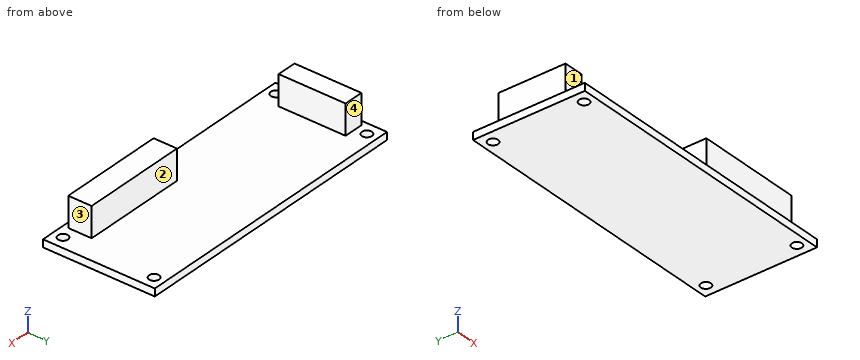
```python
from build123d import *

# Parameters (mm, degrees)
SKETCH1_W               = 91.44
SKETCH1_H               = 35.56
BOSS_EXTRUDE1_DEPTH     = 2.38125
SKETCH2_R               = 1.5875
CUT_EXTRUDE1_DEPTH      = 50.113309312
MIRROR2_COPY_1_SKETCH_R = 1.5875
MIRROR2_COPY_1_DEPTH    = 50.113309312
SKETCH3_W               = 6.208251033
SKETCH3_H               = 21.285432112
SKETCH3_W_2             = 33.591072552
SKETCH3_H_2             = 7.427728914
BOSS_EXTRUDE2_DEPTH     = 9.525


with BuildPart() as part:
    # Sketch1 → Boss-Extrude1 (new body)
    with BuildSketch(Plane.XY):
        Rectangle(SKETCH1_W, SKETCH1_H)
    extrude(amount=BOSS_EXTRUDE1_DEPTH)

    # Sketch2 → Cut-Extrude1 (cut, through all)
    with BuildSketch(Plane.XY.offset(2.38125)):
        with Locations((-41.91, 14.478)):
            Circle(SKETCH2_R)
    cut_extrude1 = extrude(amount=-CUT_EXTRUDE1_DEPTH, mode=Mode.SUBTRACT)

    # Mirror1: Cut-Extrude1 across plane
    add(cut_extrude1.mirror(Plane(origin=(0, 0, 0), x_dir=(0, 0, 1), z_dir=(1, 0, 0))), mode=Mode.SUBTRACT)

    # Mirror2: Cut-Extrude1 across plane
    add(cut_extrude1.mirror(Plane.ZX), mode=Mode.SUBTRACT)

    # Mirror2 copy 1 sketch → Mirror2 copy 1 (cut, through all)
    with BuildSketch(Plane(origin=(0, 0, 2.38125), x_dir=(-1, 0, 0), z_dir=(0, 0, 1))):
        with Locations((-41.91, 14.478)):
            Circle(MIRROR2_COPY_1_SKETCH_R)
    extrude(amount=-MIRROR2_COPY_1_DEPTH, mode=Mode.SUBTRACT)

    # Sketch3 → Boss-Extrude2 (add)
    with BuildSketch(Plane.XY.offset(2.38125)):
        with Locations((-41.018801466, 0.277154064)):
            Rectangle(SKETCH3_W, SKETCH3_H)
        with Locations((21.008278048, -12.416502065)):
            Rectangle(SKETCH3_W_2, SKETCH3_H_2)
    extrude(amount=BOSS_EXTRUDE2_DEPTH)


solid = part.part
```
Model file for the job. Use its own axes, mm. Face numbers are marked on the shaded views. A direction names the side the tool comes from. Give positions to 0.01 mm unless a question says otherwise; leave off trailing zeros. Loops run counter-clockwise (first coordinate to the right, second up) from the corner with the lowest first, then second, coordinate; pieces in that order, holes last. Notation, with made-up numbers: (-39.75, 35) -> (3.25, 35) arc R18 cw to (3.25, 45) -> close; hole circle Ø6 at (52, 53.5). An arc over 180 degrees is marked (long way). Use CSV: the item, a comma, the result in double quotes. Start each with the question number.
1) Tool access for the marked faces 1, 2, 3 and 4: list every direction of +Z, -Z, +X, -X, +Y, -Y with a clear straight run to the whole face (end or side of a thin tool).
2) Flat gauge pins, fed straight in: pin 1 Ø3 at (x, z) = (-42, 9.5) entering from +Y; pin 2 Ø12 at (x, y) = (4.5, -8.5) entering from +Z; pin 3 Ø3.5 at (y, z) = (-14, 5) entering from -X; pin 4 Ø1.9 at (x, y) = (-41.91, 14.478) entering from -Z. Where does each tip first touch, or does it go through?
3) Slice it at C-C on y = -0.5. Give the cut face in (x, z).
4) Wall check: line 1 (Y direction, x = -41.91, z = 1.7); line 2 (Z direction, x = 5, y = -7); line 3 (Y direction, x = 19, z = 4.25). Give the ranges that are in metal, low to high.
5) Slice it at D-D on x = 27. Give the cut face in (y, z), plus the area to 3 significant figures.
6) Slice it at A-A on x = 41.91. Give the cut face in (y, z).
7) Slice it at B-B on z = 8.75. Give the cut face in (x, y), plus the area to 3 significant figures.
Computed values:
1,face 1,"+Z, -X, -Y"
1,face 2,"+Z, +X, +Y"
1,face 3,"+Z, +X, +Y, -Y"
1,face 4,"+Z, +X, -X, +Y"
2,pin 1,"stops at y = 10.92"
2,pin 2,"stops at z = 11.91"
2,pin 3,"stops at x = 4.21"
2,pin 4,"passes through"
3,outline,"(-45.72, 0) -> (45.72, 0) -> (45.72, 2.38) -> (-37.91, 2.38) -> (-37.91, 11.91) -> (-44.12, 11.91) -> (-44.12, 2.38) -> (-45.72, 2.38) -> close"
4,line 1,"y = -17.78 to -16.07, -12.89 to 12.89, 16.07 to 17.78"
4,line 2,"z = 0 to 2.38"
4,line 3,"y = -16.13 to -8.7"
5,outline,"(-17.78, 0) -> (17.78, 0) -> (17.78, 2.38) -> (-8.7, 2.38) -> (-8.7, 11.91) -> (-16.13, 11.91) -> (-16.13, 2.38) -> (-17.78, 2.38) -> close"
5,area,"155 mm^2"
6,outline,"(-17.78, 0) -> (-16.07, 0) -> (-16.07, 2.38) -> (-17.78, 2.38) -> close; (-12.89, 0) -> (12.89, 0) -> (12.89, 2.38) -> (-12.89, 2.38) -> close; (16.07, 0) -> (17.78, 0) -> (17.78, 2.38) -> (16.07, 2.38) -> close"
7,outline,"(-44.12, -10.37) -> (-37.91, -10.37) -> (-37.91, 10.92) -> (-44.12, 10.92) -> close; (4.21, -16.13) -> (37.8, -16.13) -> (37.8, -8.7) -> (4.21, -8.7) -> close"
7,area,"382 mm^2"
